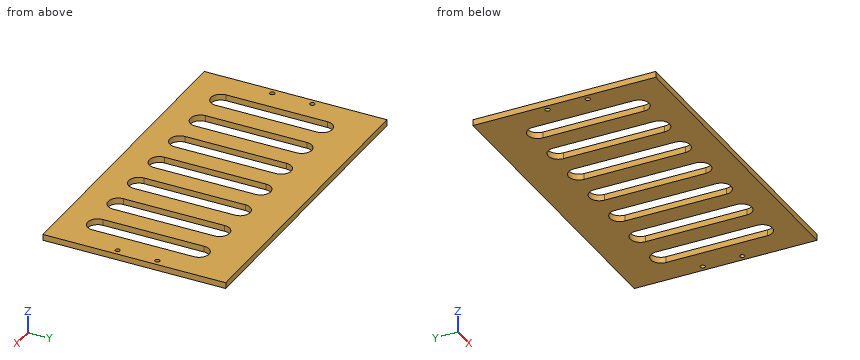
Autodesk Inventor part; units mm, degrees
ref_plane "YZ Plane" through (0, 0, 0) normal (1, 0, 0) x (0, 1, 0)
ref_plane "XZ Plane" through (0, 0, 0) normal (0, 1, 0) x (-1, 0, 0)
ref_plane "XY Plane" through (0, 0, 0) normal (0, 0, 1) x (1, 0, 0)
sketch "草图1" plane through (0, 0, 0) normal (0, 0, 1) x (1, 0, 0)
  line L0 (78.5, -47.5) -> (-78.5, -47.5)
  line L1 (-78.5, -47.5) -> (-78.5, 47.5)
  line L2 (-78.5, 47.5) -> (78.5, 47.5)
  line L3 (78.5, 47.5) -> (78.5, -47.5)
  line L4 (78.5, -47.5) -> (-78.5, 47.5) construction
  line L5 (-78.5, -47.5) -> (78.5, 47.5) construction
  point P0 (0, 0)
  dimension "d1" = 157
  dimension "d5" = 95
extrude "拉伸1" add sketch "草图1" along normal blind 3
sketch "草图2" plane through (0, 0, 3) normal (0, 0, 1) x (1, 0, 0)
  point P0 (0, 0)
sketch "草图3" plane through (0, 0, 3) normal (0, 0, 1) x (1, 0, 0)
  line L0 (-79.9462, -43.4706) -> (81.0538, -43.4706)
  line L1 (78.5, 47.5) -> (-78.5, 47.5)
  line L2 (-78.5, 47.5) -> (-78.5, -47.5)
  line L3 (-78.5, -47.5) -> (78.5, -47.5)
  line L4 (78.5, -47.5) -> (78.5, 47.5)
  point P0 (0, 0)
  point P1 (78.5, -43.4706)
  point P2 (-78.5, -43.4706)
extrude "拉伸2" cut sketch "草图3" against normal blind 10 contours L0 L4 L3 L2
sketch "草图4" plane through (0, 0, 0) normal (0, 0, -1) x (-1, 0, 0)
  circle A0 centre (-75.5, 11.9042) radius 1.2
  ellipse E0 centre (-75.5, -7.8467) end of major axis (-76.7, -7.8467) minor radius 1.1265
  circle A1 centre (75.5, 11.9042) radius 1.2
  circle A2 centre (75.5, -8.0958) radius 1.2
  point P0 (0, 0)
extrude "拉伸3" cut sketch "草图4" against normal blind 10
sketch "草图5" plane through (0, 0, 3) normal (0, 0, 1) x (1, 0, 0)
  line L0 (-60, 24.7542) -> (-60, -25.6955) construction
  line L1 (-65, 24.7542) -> (-65, -25.6955)
  line L2 (-55, -25.6955) -> (-55, 24.7542)
  arc A0 (-55, 24.7542) -> (-65, 24.7542) centre (-60, 24.7542) ccw
  arc A1 (-65, -25.6955) -> (-55, -25.6955) centre (-60, -25.6955) ccw
  line L3 (-78.5, -43.4706) -> (78.5, -43.4706)
  line L4 (-40, 24.7542) -> (-40, -25.6955) construction
  line L5 (-45, 24.7542) -> (-45, -25.6955)
  line L6 (-35, -25.6955) -> (-35, 24.7542)
  arc A2 (-35, 24.7542) -> (-45, 24.7542) centre (-40, 24.7542) ccw
  arc A3 (-45, -25.6955) -> (-35, -25.6955) centre (-40, -25.6955) ccw
  line L7 (-20, 24.7542) -> (-20, -25.6955) construction
  line L8 (-25, 24.7542) -> (-25, -25.6955)
  line L9 (-15, -25.6955) -> (-15, 24.7542)
  arc A4 (-15, 24.7542) -> (-25, 24.7542) centre (-20, 24.7542) ccw
  arc A5 (-25, -25.6955) -> (-15, -25.6955) centre (-20, -25.6955) ccw
  line L10 (0, 24.7542) -> (0, -25.6955) construction
  line L11 (-5, 24.7542) -> (-5, -25.6955)
  line L12 (5, -25.6955) -> (5, 24.7542)
  arc A6 (5, 24.7542) -> (-5, 24.7542) centre (0, 24.7542) ccw
  arc A7 (-5, -25.6955) -> (5, -25.6955) centre (0, -25.6955) ccw
  line L13 (20, 24.7542) -> (20, -25.6955) construction
  line L14 (15, 24.7542) -> (15, -25.6955)
  line L15 (25, -25.6955) -> (25, 24.7542)
  arc A8 (25, 24.7542) -> (15, 24.7542) centre (20, 24.7542) ccw
  arc A9 (15, -25.6955) -> (25, -25.6955) centre (20, -25.6955) ccw
  line L16 (40, 24.7542) -> (40, -25.6955) construction
  line L17 (35, 24.7542) -> (35, -25.6955)
  line L18 (45, -25.6955) -> (45, 24.7542)
  arc A10 (45, 24.7542) -> (35, 24.7542) centre (40, 24.7542) ccw
  arc A11 (35, -25.6955) -> (45, -25.6955) centre (40, -25.6955) ccw
  line L19 (60, 24.7542) -> (60, -25.6955) construction
  line L20 (55, 24.7542) -> (55, -25.6955)
  line L21 (65, -25.6955) -> (65, 24.7542)
  arc A12 (65, 24.7542) -> (55, 24.7542) centre (60, 24.7542) ccw
  arc A13 (55, -25.6955) -> (65, -25.6955) centre (60, -25.6955) ccw
  line L22 (80, 24.7542) -> (80, -25.6955) construction
  line L23 (75, 24.7542) -> (75, -25.6955)
  line L24 (85, -25.6955) -> (85, 24.7542)
  arc A14 (85, 24.7542) -> (75, 24.7542) centre (80, 24.7542) ccw
  arc A15 (75, -25.6955) -> (85, -25.6955) centre (80, -25.6955) ccw
  line L25 (100, 24.7542) -> (100, -25.6955) construction
  line L26 (95, 24.7542) -> (95, -25.6955)
  line L27 (105, -25.6955) -> (105, 24.7542)
  arc A16 (105, 24.7542) -> (95, 24.7542) centre (100, 24.7542) ccw
  arc A17 (95, -25.6955) -> (105, -25.6955) centre (100, -25.6955) ccw
  line L28 (120, 24.7542) -> (120, -25.6955) construction
  line L29 (115, 24.7542) -> (115, -25.6955)
  line L30 (125, -25.6955) -> (125, 24.7542)
  arc A18 (125, 24.7542) -> (115, 24.7542) centre (120, 24.7542) ccw
  arc A19 (115, -25.6955) -> (125, -25.6955) centre (120, -25.6955) ccw
  line L31 (-78.5, 47.5) -> (-78.5, -43.4706)
  line L32 (78.5, -43.4706) -> (78.5, 47.5)
  point P0 (0, 0)
  point P1 (-60, -0.4706)
  point P2 (-40, -0.4706)
  point P3 (-20, -0.4706)
  point P4 (0, -0.4706)
  point P5 (20, -0.4706)
  point P6 (40, -0.4706)
  point P7 (60, -0.4706)
  point P8 (80, -0.4706)
  point P9 (100, -0.4706)
  point P10 (120, -0.4706)
  dimension "d10" = 10
  dimension "d11" = 43
  dimension "d17" = 20
  dimension "d21" = 13.5
  dimension "d22" = 13.5
extrude "拉伸4" cut sketch "草图5" against normal blind 73.5 contours A0 L2 A1 L1 | A2 L6 A3 L5 | A4 L9 A5 L8 | A6 L12 A7 L11 | A8 L15 A9 L14 | A10 L18 A11 L17 | A12 L21 A13 L20
properties part number "后板3"
Can you work these out from the model? Positions are in its coordinate system, mm. Coordinates: 2 decimals unless noted, no trailing zeros. Order: outer loops, then holes, each group sorted by start corner. A loop starts at its lowest first (then second) coordinate and runs counter-clockwise, first axis right, second up.
1. I need wall thicknesses on line 1 (Y direction, x = -75.5, z = 1.2); line 2 (Y direction, x = 75.5, z = 2.35); line 3 (Y direction, x = -60.5, z = 0.4). Which ranges of each line are inside material? Lowest first, please.
2. If we section it at A-A (x = -20): Please give me the cut outline in (y, z).
3. I'm going to push a flat-ended pin straight in: pin 1 (1.4 mm diameter, centred on x = 75.5, y = 11.9, fed in from +Z). Where does the tip first touch, or does it pass through?
4. If we section it at B-B (y = 17): Give the number of separate pieces and of enclosed holes in the cut face, then the cut area to 3 significant figures.
Entries:
1. line 1: y = -43.47 to -9.3, -6.9 to 10.7, 13.1 to 47.5
1. line 2: y = -43.47 to -8.97, -6.72 to 10.7, 13.1 to 47.5
1. line 3: y = -43.47 to -30.67, 29.73 to 47.5
2. outline: (-43.47, 0) - (-30.7, 0) - (-30.7, 3) - (-43.47, 3) - close; (29.75, 0) - (47.5, 0) - (47.5, 3) - (29.75, 3) - close
3. pin 1: passes through
4. separate pieces: 8
4. enclosed holes: 0
4. area: 261 mm2
